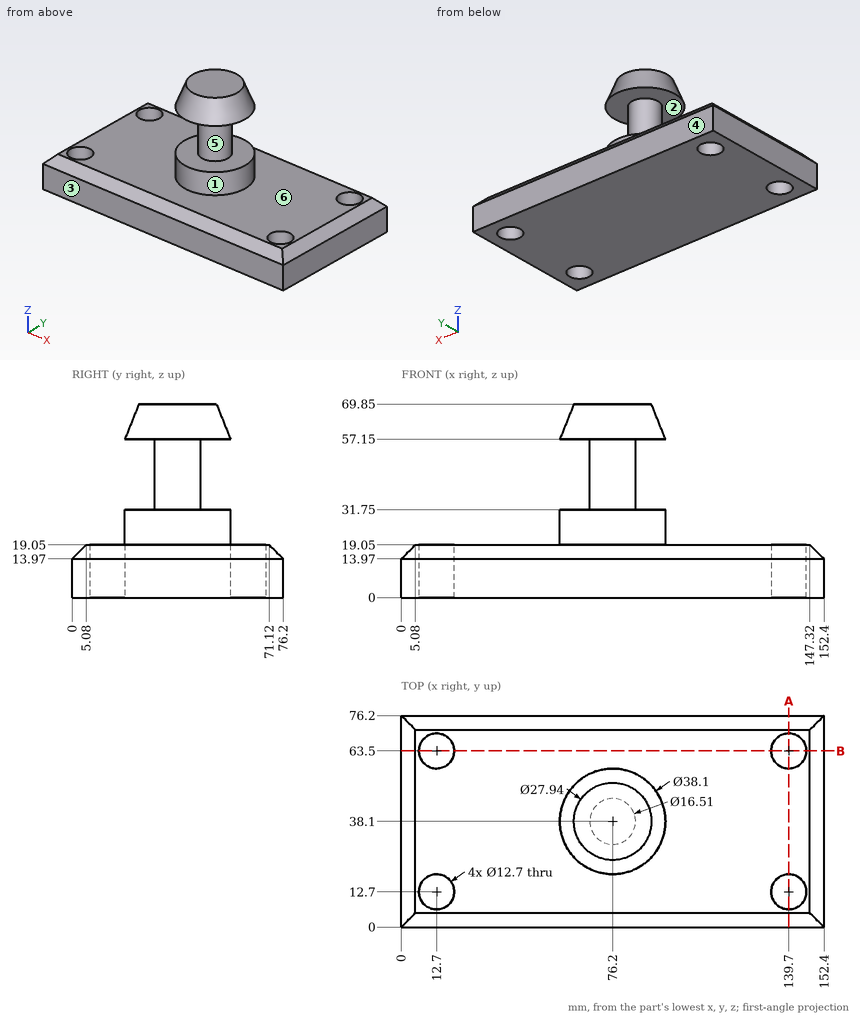
Geometry check sheet. Reference: drawing and pictorial views, mm from the part's lowest x, y, z. A direction names the side the tool comes from. Give positions to 0.01 mm unless a question says otherwise; leave off trailing zeros. Write each loop counter-clockwise with the first axis right and the second up, starting at its lowest first coordinate (ties: lowest second). Pieces come first, ordered by that corner, then holes. Notation, with made-up numbers: M 84.25,-32 L 134.25,-32 A26 ccw 134.25,2 Z; hole C 61.25,-27.5 d2. An arc over 180 degrees is marked long. Answer as CSV lines item,"result". Start each with the question number.
Q1. Material ranges on L1, parallel to X at y = 63.5, z = 4; L2, parallel to Y at x = 139.7, z = 6.25; L3, parallel to Z at x = 91, y = 61, recorded low to high.
Q2. Go/stop test with flat-tipped pins: pin 1 (1 mm diameter, centred on x = 39, y = 56, fed in from +Z); pin 2 (1.5 mm diameter, centred on y = 51, z = 20.5, fed in from +X); pin 3 (5 mm diameter, centred on y = 35, z = 21.5, fed in from +X); pin 4 (7.5 mm diameter, centred on x = 12.7, y = 12.7, fed in from -Z). Record where each tip stops, or that it passes through.
Q3. Tool access check on the marked faces 1, 2 and 3. Record the directions out of +Z, -Z, +X, -X, +Y, -Y that give a thin tool (end or side, any length) a straight path to the whole face; none if there is none.
Q4. Section check A-A, the plane x = 139.7. Record the cut outline in (y, z).
Q5. Release check for a two-part mould opening along Z. For the marked faces 4, 5 and 6 record: pulls with the +Z half, pulls with the -Z half, needs draft (parallel to the pull), parting line crosses it, or undercut.
Q6. Section check B-B, the plane y = 63.5. Record the cut outline in (x, z).
Geometry says:
1,L1,"0 to 6.35, 19.05 to 133.35, 146.05 to 152.4"
1,L2,"0 to 6.35, 19.05 to 57.15, 69.85 to 76.2"
1,L3,"0 to 19.05"
2,pin 1,"z = 19.05"
2,pin 2,"x = 90.87"
2,pin 3,"x = 147.37"
2,pin 4,"through"
3,face 1,"+Z"
3,face 2,"none"
3,face 3,"+Z, -Z, +X, -X, -Y"
4,outline,"M 0,0 L 6.35,0 L 6.35,19.05 L 5.08,19.05 L 0,13.97 Z; M 19.05,0 L 57.15,0 L 57.15,19.05 L 19.05,19.05 Z; M 69.85,0 L 76.2,0 L 76.2,13.97 L 71.12,19.05 L 69.85,19.05 Z"
5,face 4,"needs draft"
5,face 5,"undercut"
5,face 6,"pulls with the +Z half"
6,outline,"M 0,0 L 6.35,0 L 6.35,19.05 L 5.08,19.05 L 0,13.97 Z; M 19.05,0 L 133.35,0 L 133.35,19.05 L 19.05,19.05 Z; M 146.05,0 L 152.4,0 L 152.4,13.97 L 147.32,19.05 L 146.05,19.05 Z"
